from build123d import *

# Parameters (mm, degrees)
SKETCH1_R           = 15
BOSS_EXTRUDE1_DEPTH = 30


with BuildPart() as part:
    # Sketch1 → Boss-Extrude1 (new body)
    with BuildSketch(Plane.XY):
        with BuildLine():
            Line((-1.85478455, 19.913808633), (77.446717813, 27.3))
            Line((77.446717813, 27.3), (171.085265534, 19.938479729))
            ThreePointArc((171.085265534, 19.938479729), (189.455188028, -1.581002183), (167.923261894, -19.936336862))
            Line((167.923261894, -19.936336862), (77.446717813, -12.7))
            Line((77.446717813, -12.7), (1.900000117, -19.909545438))
            ThreePointArc((1.900000117, -19.909545438), (-19.91168987, -1.877393544), (-1.85478455, 19.913808633))
        make_face()
        with Locations((77.446717813, 7.3)):
            Circle(SKETCH1_R, mode=Mode.SUBTRACT)
        with Locations((169.517775155, 0)):
            Circle(SKETCH1_R, mode=Mode.SUBTRACT)
        Circle(SKETCH1_R, mode=Mode.SUBTRACT)
    extrude(amount=BOSS_EXTRUDE1_DEPTH)


solid = part.part
Geometry: final body of the model. Coordinates: model frame, mm. A direction names the side the tool comes from. Give positions to 0.01 mm unless a question says otherwise; leave off trailing zeros. Write each loop counter-clockwise with the first axis right and the second up, starting at its lowest first coordinate (ties: lowest second). Pieces come first, ordered by that corner, then holes. Notation, with made-up numbers: (-24.75, -27) - (29.25, -27) arc R20 cw to (29.25, -5) - close; hole circle Ø2 at (3, 56.25). An arc over 180 degrees is marked (long way). Return JSON: item names as keys, results as strings. Group by question number.
1) Mould query, pull axis Y, two halves, no side actions, for faces 3 (the cylindrical face through (62.46, 7.96, 14.79)), 4 (the flat face through (123.61, 23.67, 14.79)), 5 (the flat face through (40.202, -16.254, 14.79)), 6 (the flat face through (86, -7, 0)). Classes: released by +Y, released by -Y, zero draft, split by the parting line, or undercut.
2) Section D-D on x = 0. Return the cut outline in (y, z).
3) Line query: line 1 (X direction, y = -12, z = 25); line 2 (X direction, y = -10.5, z = 27.75); line 3 (X direction, y = 9, z = 16). Output: solid intervals per line, ascending.
4) Set-up query: faces 1 (the flat face through (123.32, -16.37, 14.79)), 2 (the flat face through (37.241, 23.555, 14.79)). Return all of +Z, -Z, +X, -X, +Y, -Y with unobstructed straight access to the full face (end or side cutting, diameter ignored); none if empty.
5) Section B-B on y = 5. Return the cut outline in (x, z), plus the area to 3 significant figures.
6) Section A-A on z = 17.5. Return the cut outline in (x, y), plus the area to 3 significant figures.
7) Section C-C on x = 71. Return the cut outline in (y, z).
8) First-contact query: P1, Ø18, axis at x = 169.52, y = 0, coming from the +Z side; P2, Ø1.5, axis at y = 13, z = 15, coming from the -X side; P3, Ø5, axis at x = 37.5, z = 25, coming from the -Y side; P4, Ø1.5, axis at x = 71, z = 8.5, coming from the -Y side. Flat tips, straight axial feed; report the tip coordinate or a pass-through.
Filled in:
{
 "1": {"face 3": "undercut", "face 4": "released by +Y", "face 5": "released by -Y", "face 6": "zero draft"},
 "2": {"outline": "(-20, 0) - (-15, 0) - (-15, 30) - (-20, 30) - close; (15, 0) - (20.09, 0) - (20.09, 30) - (15, 30) - close"},
 "3": {"line 1": "x = -16 to -9, 9 to 160.52, 178.52 to 185.52", "line 2": "x = -17.02 to -10.71, 10.71 to 158.81, 180.23 to 186.54", "line 3": "x = -17.86 to -12, 12 to 62.54, 92.35 to 157.52, 181.52 to 187.38"},
 "4": {"face 1": "+Z, -Z, -Y", "face 2": "+Z, -Z, -X, +Y"},
 "5": {"outline": "(-19.36, 0) - (-14.14, 0) - (-14.14, 30) - (-19.36, 30) - close; (14.14, 0) - (62.62, 0) - (62.62, 30) - (14.14, 30) - close; (92.27, 0) - (155.38, 0) - (155.38, 30) - (92.27, 30) - close; (183.66, 0) - (188.88, 0) - (188.88, 30) - (183.66, 30) - close", "area": "3,660 mm^2"},
 "6": {"outline": "(-1.85, 19.91) arc R20 ccw to (1.9, -19.91) - (77.45, -12.7) - (167.92, -19.94) arc R20 ccw to (171.09, 19.94) - (77.45, 27.3) - close; hole circle Ø30 at (0, 0); hole circle Ø30 at (77.45, 7.3); hole circle Ø30 at (169.52, 0)", "area": "5,930 mm^2"},
 "7": {"outline": "(-13.32, 0) - (-6.24, 0) - (-6.24, 30) - (-13.32, 30) - close; (20.84, 0) - (26.7, 0) - (26.7, 30) - (20.84, 30) - close"},
 "8": {"P1": "passes through", "P2": "stops at x = -15.81", "P3": "stops at y = -16.75", "P4": "stops at y = -13.39"}
}
